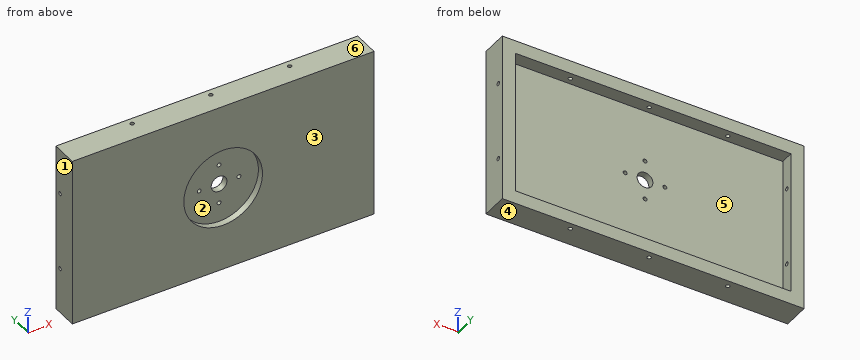
```python
from build123d import *

# Parameters (mm, degrees)
SKETCH1_W           = 210
SKETCH1_H           = 110
BOSS_EXTRUDE1_DEPTH = 10
CUT_EXTRUDE1_DEPTH  = 5
SKETCH3_R           = 1.5
CUT_EXTRUDE2_DEPTH  = 5
SKETCH4_R           = 6
CUT_EXTRUDE3_DEPTH  = 5
SKETCH5_R           = 30
CUT_EXTRUDE4_DEPTH  = 5
SKETCH10_W          = 210
SKETCH10_H          = 110
BOSS_EXTRUDE2_DEPTH = 20
SKETCH11_R          = 1.5
CUT_EXTRUDE6_DEPTH  = 300
SKETCH12_R          = 1.5
CUT_EXTRUDE7_DEPTH  = 300


with BuildPart() as part:
    # Sketch1 → Boss-Extrude1 (new body)
    with BuildSketch(Plane(origin=(0, 0, 0), x_dir=(1, 0, 0), z_dir=(0, 1, 0))):
        with Locations((105, -55)):
            Rectangle(SKETCH1_W, SKETCH1_H)
    extrude(amount=BOSS_EXTRUDE1_DEPTH)

    # Sketch2 → Cut-Extrude1 (cut)
    with BuildSketch(Plane(origin=(0, 0, 0), x_dir=(-1, 0, 0), z_dir=(0, -1, 0))):
        with BuildLine():
            ThreePointArc((-130, -55), (-105, -80), (-80, -55))
            Line((-80, -55), (-130, -55))
        make_face()
        with BuildLine():
            Line((-130, -55), (-80, -55))
            ThreePointArc((-80, -55), (-105, -30), (-130, -55))
        make_face()
    extrude(amount=-CUT_EXTRUDE1_DEPTH, mode=Mode.SUBTRACT)

    # Sketch3 → Cut-Extrude2 (cut)
    with BuildSketch(Plane(origin=(0, 5, 0), x_dir=(-1, 0, 0), z_dir=(0, -1, 0))):
        with Locations(Location((-105, -70.12891571, 0), (0, 0, 90))):
            Circle(SKETCH3_R)
        with Locations(Location((-120.12891571, -55, 0), (0, 0, 90))):
            Circle(SKETCH3_R)
        with Locations(Location((-105, -39.87108429, 0), (0, 0, 90))):
            Circle(SKETCH3_R)
        with Locations(Location((-89.87108429, -55, 0), (0, 0, 90))):
            Circle(SKETCH3_R)
    extrude(amount=-CUT_EXTRUDE2_DEPTH, mode=Mode.SUBTRACT)

    # Sketch4 → Cut-Extrude3 (cut)
    with BuildSketch(Plane(origin=(0, 5, 0), x_dir=(-1, 0, 0), z_dir=(0, -1, 0))):
        with Locations(Location((-105, -55, 0), (0, 0, 90))):
            Circle(SKETCH4_R)
    extrude(amount=-CUT_EXTRUDE3_DEPTH, mode=Mode.SUBTRACT)

    # Sketch5 → Cut-Extrude4 (cut)
    with BuildSketch(Plane(origin=(0, 0, 0), x_dir=(-1, 0, 0), z_dir=(0, -1, 0))):
        with Locations(Location((-105, -55, 0), (0, 0, 90))):
            Circle(SKETCH5_R)
    extrude(amount=-CUT_EXTRUDE4_DEPTH, mode=Mode.SUBTRACT)

    # Sketch10 → Boss-Extrude2 (add)
    with BuildSketch(Plane(origin=(0, 0, 0), x_dir=(-1, 0, 0), z_dir=(0, -1, 0))):
        Polygon((10, -110), (10, 10), (-220, 10), (-220, -120), (10, -120), align=None)
        with Locations((-105, -55)):
            Rectangle(SKETCH10_W, SKETCH10_H, mode=Mode.SUBTRACT)
    extrude(amount=-BOSS_EXTRUDE2_DEPTH)

    # Sketch11 → Cut-Extrude6 (cut)
    with BuildSketch(Plane.ZY.offset(10)):
        with Locations((25, 15)):
            Circle(SKETCH11_R)
        with Locations((85, 15)):
            Circle(SKETCH11_R)
    extrude(amount=-CUT_EXTRUDE6_DEPTH, mode=Mode.SUBTRACT)

    # Sketch12 → Cut-Extrude7 (cut)
    with BuildSketch(Plane.XY.offset(120)):
        with Locations(Location((45, 15, 0), (0, 0, 180))):
            Circle(SKETCH12_R)
        with Locations(Location((165, 15, 0), (0, 0, 180))):
            Circle(SKETCH12_R)
        with Locations(Location((105, 15, 0), (0, 0, 180))):
            Circle(SKETCH12_R)
    extrude(amount=-CUT_EXTRUDE7_DEPTH, mode=Mode.SUBTRACT)


solid = part.part
```
Geometry check sheet. Reference: the model listing, model coordinates, mm. Face numbers are marked on the shaded views. A direction names the side the tool comes from. Round coordinates to 2 decimals unless told otherwise and drop trailing zeros. Order: outer loops, then holes, each group sorted by start corner. A loop starts at its lowest first (then second) coordinate and runs counter-clockwise, first axis right, second up. Notation, with made-up numbers: M 52.25,50.5 L 97.25,50.5 A30 ccw 97.25,74.5 Z; hole C 5.25,75 d6. An arc over 180 degrees is marked long. Answer as CSV lines item,"result".
1) Thickness scan on probe 1 along X at (y, z) = (7.45, 55); probe 2 along X at (y, z) = (15, -6); probe 3 along Y at (x, z) = (165, -3). Record the ranges inside material, lowest first. Write a range as [from, to].
Entries:
probe 1,"[-10, 88.37], [91.37, 99], [111, 118.63], [121.63, 220]"
probe 2,"[-10, 43.5], [46.5, 103.5], [106.5, 163.5], [166.5, 220]"
probe 3,"[0, 13.5], [16.5, 20]"
2) Mould release check, pull along Z, two halves, no side actions. Record for the marked faces 3, 4, 5 and 6: +Z half, -Z half, draft (parallel to the pull), parting line (faces both ways), or undercut.
Entries:
face 3,"draft"
face 4,"-Z half"
face 5,"undercut"
face 6,"+Z half"
3) Sectioned sample at B-B on x = 169.5. Record the cut outline in (y, z).
Entries:
outline,"M 0,-10 L 20,-10 L 20,0 L 10,0 L 10,110 L 20,110 L 20,120 L 0,120 Z"
4) Sectioned sample at A-A on z = 18. Record the cut outline in (x, y).
Entries:
outline,"M -10,0 L 220,0 L 220,20 L 210,20 L 210,10 L 0,10 L 0,20 L -10,20 Z"
5) Tool access check on the marked faces 1 and 2. Record the directions out of +Z, -Z, +X, -X, +Y, -Y that give a thin tool (end or side, any length) a straight path to the whole face; none if there is none.
Entries:
face 1,"+Z, -Z, -X, +Y, -Y"
face 2,"-Y"
6) Gauge pin test, flat ends, axial feed: pin 1 Ø2.5 at (x, z) = (120.13, 55) entering from -Y; pin 2 Ø1.5 at (x, z) = (120, 60) entering from -Y. Record the tip position at first contact, or that the pin passes through.
Entries:
pin 1,"through"
pin 2,"y = 5"
